Verification items for the finished model (mm, model axes). A direction names the side the tool comes from. Give positions to 0.01 mm unless a question says otherwise; leave off trailing zeros. Order: outer loops, then holes, each group sorted by start corner. A loop starts at its lowest first (then second) coordinate and runs counter-clockwise, first axis right, second up.
(1) Sectioned sample at C-C on x = 0. Record the cut outline in (y, z).
(2) Gauge pin test, flat ends, axial feed: pin 1 (2 mm diameter, centred on y = 16.5, z = -0.5, fed in from +X); pin 2 (2 mm diameter, centred on x = -10, y = 18.5, fed in from +Z); pin 3 (2.5 mm diameter, centred on y = 10, z = 1, fed in from -X); pin 4 (4 mm diameter, centred on x = -24.5, z = -1, fed in from +Y). Record the tip position at first contact, or that the pin passes through.
(3) Mould release check, pull along X, two halves, no side actions. Record for faces 1 (the face through (-20, 0, 2)), 2 (the face through (-14.678, 10, 0)), 3 (the face through (-10.678, 7, 0)): pulls with the +X half, pulls with the -X half, needs draft (parallel to the pull), parting line crosses it, or undercut.
(4) Scan lines: L1, parallel to X at y = 3.05, z = 0; L2, parallel to X at y = 5, z = 2.5; L3, parallel to X at y = 2, z = -3.5. Record each from-to range of solid material in increasing order.
(5) Sectioned sample at D-D on y = 19. Record the cut outline in (x, z), plus the area to 3 significant figures.
(6) Sectioned sample at A-A on y = 7.5. Record the cut outline in (x, z), plus the area to 3 significant figures.
(7) Sectioned sample at B-B on z = 0. Record the cut outline in (x, y) (1 decimal).
(8) Access from +Z, -Z, +X, -X, +Y, -Y to the whole of each face (thin tool, end or side, straight path). Record for faces 4 (the face through (10.678, 8, 0)), 5 (the face through (20, 4, 2)), 6 (the face through (-20, 4, 2)).
```python
from build123d import *

# Parameters (mm, degrees)
STRAP_DEPTH        = 4
EAR_HOLES_M4_START = -0.5
SKETCH2_R          = 2.25
EAR_HOLES_M4_DEPTH = 5


with BuildPart() as part:
    # Sketch1 → Strap (new, symmetric)
    with BuildSketch(Plane.XY):
        with BuildLine():
            Line((-28.6775, 0), (-10.6775, 0))
            Line((-10.6775, 0), (-10.6775, 15))
            ThreePointArc((-10.6775, 15), (0, 25.6775), (10.6775, 15))
            Line((10.6775, 15), (10.6775, 0))
            Line((10.6775, 0), (28.6775, 0))
            Line((28.6775, 0), (28.6775, 4))
            Line((28.6775, 4), (14.6775, 4))
            Line((14.6775, 4), (14.6775, 15))
            ThreePointArc((14.6775, 15), (0, 29.6775), (-14.6775, 15))
            Line((-14.6775, 15), (-14.6775, 4))
            Line((-14.6775, 4), (-28.6775, 4))
            Line((-28.6775, 4), (-28.6775, 0))
        make_face()
    extrude(amount=STRAP_DEPTH, both=True)

    # Sketch2 → Ear_Holes_M4 (cut)
    with BuildSketch(Plane(origin=(0, 0, 0), x_dir=(1, 0, 0), z_dir=(0, 1, 0)).offset(EAR_HOLES_M4_START)):
        with Locations(Location((-21.6775, 0, 0), (0, 0, 90))):
            Circle(SKETCH2_R)
        with Locations(Location((21.6775, 0, 0), (0, 0, 90))):
            Circle(SKETCH2_R)
    extrude(amount=EAR_HOLES_M4_DEPTH, mode=Mode.SUBTRACT)


solid = part.part
```
Ans:
1. outline: (25.68, -4) - (29.68, -4) - (29.68, 4) - (25.68, 4) - close
2. pin 1: stops at x = 14.67
2. pin 2: stops at z = 4
2. pin 3: stops at x = -14.68
2. pin 4: stops at y = 4
3. face 1: needs draft
3. face 2: pulls with the -X half
3. face 3: undercut
4. L1: x = -28.68 to -23.93, -19.43 to -10.68, 10.68 to 19.43, 23.93 to 28.68
4. L2: x = -14.68 to -10.68, 10.68 to 14.68
4. L3: x = -28.68 to -10.68, 10.68 to 28.68
5. outline: (-14.12, -4) - (-9.9, -4) - (-9.9, 4) - (-14.12, 4) - close; (9.9, -4) - (14.12, -4) - (14.12, 4) - (9.9, 4) - close
5. area: 67.6 mm2
6. outline: (-14.68, -4) - (-10.68, -4) - (-10.68, 4) - (-14.68, 4) - close; (10.68, -4) - (14.68, -4) - (14.68, 4) - (10.68, 4) - close
6. area: 64.0 mm2
7. outline: (-28.7, 0) - (-23.9, 0) - (-23.9, 4) - (-28.7, 4) - close; (-19.4, 0) - (-10.7, 0) - (-10.7, 15) arc R10.7 cw to (10.7, 15) - (10.7, 0) - (19.4, 0) - (19.4, 4) - (14.7, 4) - (14.7, 15) arc R14.7 ccw to (-14.7, 15) - (-14.7, 4) - (-19.4, 4) - close; (23.9, 0) - (28.7, 0) - (28.7, 4) - (23.9, 4) - close
8. face 4: +Z, -Z, -Y
8. face 5: +Z, -Z, +X, +Y
8. face 6: +Z, -Z, -X, +Y
